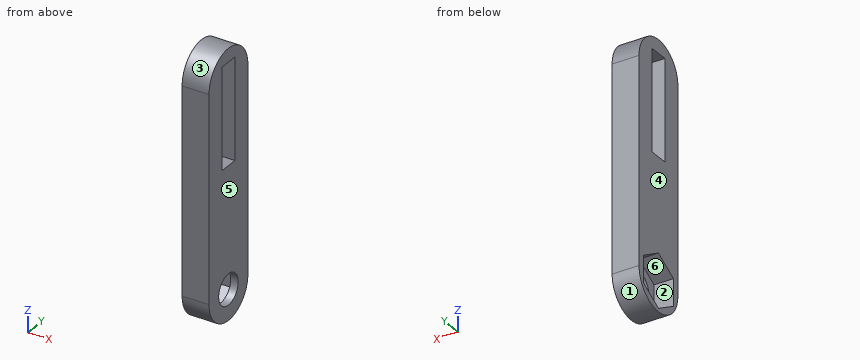
```python
from build123d import *

# Parameters (mm, degrees)
BOSS_EXTRUDE1_DEPTH      = 3.175
M3_CLEARANCE_HOLE1_D     = 3.6
M3_CLEARANCE_HOLE1_DEPTH = 7.62
M3_CLEARANCE_HOLE1_TIP   = 1.081549114
SKETCH9_W                = 11.90625
SKETCH9_H                = 2.38125
CUT_EXTRUDE1_DEPTH       = 17.360887498
CUT_EXTRUDE2_DEPTH       = 2.286


with BuildPart() as part:
    # Sketch1 → Boss-Extrude1 (new body)
    with BuildSketch(Plane(origin=(0, 0, 0), x_dir=(0, 0, -1), z_dir=(1, 0, 0))):
        with BuildLine():
            Line((-12.075480167, 3.571875), (12.075480167, 3.571875))
            ThreePointArc((12.075480167, 3.571875), (15.647355167, 0), (12.075480167, -3.571875))
            Line((12.075480167, -3.571875), (-12.075480167, -3.571875))
            ThreePointArc((-12.075480167, -3.571875), (-15.647355167, 0), (-12.075480167, 3.571875))
        make_face()
    extrude(amount=BOSS_EXTRUDE1_DEPTH)

    # M3 Clearance Hole1
    with Locations(Plane.ZY):
        with Locations((-12.075480167, 0)):
            Hole(M3_CLEARANCE_HOLE1_D / 2, depth=M3_CLEARANCE_HOLE1_DEPTH)
            with Locations((0, 0, -(M3_CLEARANCE_HOLE1_DEPTH + M3_CLEARANCE_HOLE1_TIP / 2))):  # 118° drill point
                Cone(0, M3_CLEARANCE_HOLE1_D / 2, M3_CLEARANCE_HOLE1_TIP, mode=Mode.SUBTRACT)

    # Sketch9 → Cut-Extrude1 (cut, through all)
    with BuildSketch(Plane.ZY):
        with Locations((8.106730167, 0)):
            Rectangle(SKETCH9_W, SKETCH9_H)
    extrude(amount=-CUT_EXTRUDE1_DEPTH, mode=Mode.SUBTRACT)

    # Sketch10 → Cut-Extrude2 (cut)
    with BuildSketch(Plane.ZY):
        Polygon((-10.48436056, -2.7559), (-8.893240953, 0), (-10.48436056, 2.7559), (-13.666599774, 2.7559), (-15.257719381, 0), (-13.666599774, -2.7559), align=None)
    extrude(amount=-CUT_EXTRUDE2_DEPTH, mode=Mode.SUBTRACT)


solid = part.part
```
Can you work these out from the model? Positions are in its coordinate system, mm. Face numbers are marked on the shaded views. A direction names the side the tool comes from. Coordinates: 2 decimals unless noted, no trailing zeros. Loops run counter-clockwise (first coordinate to the right, second up) from the corner with the lowest first, then second, coordinate; pieces in that order, holes last. Notation, with made-up numbers: (-21.75, 9.25) -> (3.25, 9.25) arc R34 ccw to (3.25, 45.25) -> close; hole circle Ø4 at (-32.5, 78.5). An arc over 180 degrees is marked (long way). Put each result on its own line as item: value. Start each with the question number.
Q1. For the marked faces 5 and 6, which set-ups out of +Z, -Z, +X, -X, +Y, -Y let a thin tool reach every point of the face, with its end or its side?
Q2. I want a section at C-C (y = -0.5). Write out the boundary of the cut face in (x, z) (3 decimals).
Q3. I'm going to push flat-ended pins straight in: P1, Ø1.1, axis at x = 1.5, z = -13, coming from the -Y side; P2, Ø1.9, axis at x = 1, y = -0.5, coming from the +Z side. Where does each tip first touch, or does it pass through?
Q4. I want a section at A-A (z = 7). Write out the boundary of the cut face in (x, y) (3 decimals), plus the area to 3 significant figures.
Q5. I want a section at B-B (x = 1.75). Write out the boundary of the cut face in (y, z), plus the area to 3 significant figures.
Q6. If I drill on line 1 (Y direction, x = 0.85, z = 4); line 2 (Z direction, x = 1.6, y = 1); line 3 (Y direction, x = 2, z = -12), over which ranges is the centre line in solid material (lowest first)? Write a range as [from, to].
Q7. Thinking about a two-plate mould opening in Z: for the marked faces 1, 2, 3 and 4, which applies, pulls with the +Z half, pulls with the -Z half, needs draft (parallel to the pull), parting line crosses it, or undercut?
Q8. I want a section at D-D (z = 13). Write out the boundary of the cut face in (x, y) (3 decimals), plus the area to 3 significant figures.
Taken from the geometry:
1. face 5: +Z, -Z, +X, +Y, -Y
1. face 6: -X
2. outline: (0, -15.612) -> (3.175, -15.612) -> (3.175, -13.805) -> (2.286, -13.805) -> (2.286, -14.969) -> (0, -14.969) -> close; (0, -9.182) -> (2.286, -9.182) -> (2.286, -10.346) -> (3.175, -10.346) -> (3.175, 2.154) -> (0, 2.154) -> close; (0, 14.06) -> (3.175, 14.06) -> (3.175, 15.612) -> (0, 15.612) -> close
3. P1: stops at y = -3.55
3. P2: stops at z = 15.65
4. outline: (0, -3.572) -> (3.175, -3.572) -> (3.175, -1.191) -> (0, -1.191) -> close; (0, 1.191) -> (3.175, 1.191) -> (3.175, 3.572) -> (0, 3.572) -> close
4. area: 15.1 mm2
5. outline: (-3.57, -12.08) arc R3.57 ccw to (3.57, -12.08) -> (3.57, 12.08) arc R3.57 ccw to (-3.57, 12.08) -> close; hole (-2.76, -13.67) -> (0, -15.26) -> (2.76, -13.67) -> (2.76, -10.48) -> (0, -8.89) -> (-2.76, -10.48) -> close; hole (-1.19, 2.15) -> (1.19, 2.15) -> (1.19, 14.06) -> (-1.19, 14.06) -> close
5. area: 158 mm2
6. line 1: y = [-3.57, -1.19], [1.19, 3.57]
6. line 2: z = [-15.5, -14.68], [-9.47, 2.15], [14.06, 15.5]
6. line 3: y = [-3.57, -2.76], [2.76, 3.57]
7. face 1: pulls with the -Z half
7. face 2: undercut
7. face 3: pulls with the +Z half
7. face 4: needs draft
8. outline: (0, -3.45) -> (3.175, -3.45) -> (3.175, -1.191) -> (0, -1.191) -> close; (0, 1.191) -> (3.175, 1.191) -> (3.175, 3.45) -> (0, 3.45) -> close
8. area: 14.3 mm2
